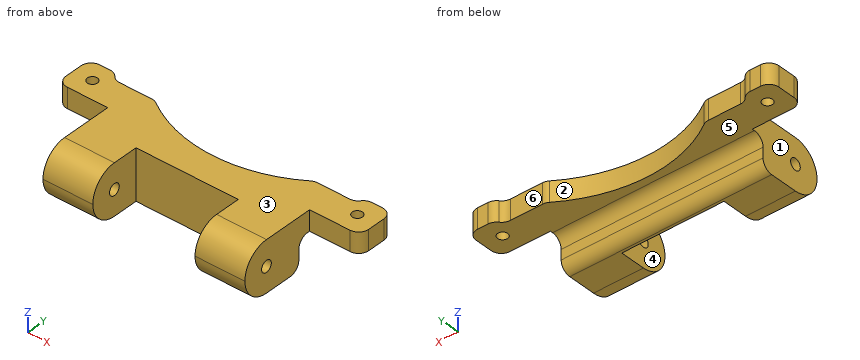
from build123d import *

# Parameters (mm, degrees)
SKETCH1_W           = 80
SKETCH1_H           = 20
BOSS_EXTRUDE1_DEPTH = 30
SKETCH2_W           = 40.5
SKETCH2_H           = 20
CUT_EXTRUDE1_DEPTH  = 20
SKETCH3_R           = 2.25
CUT_EXTRUDE2_DEPTH  = 88.749643874
FILLET1_R           = 10
SKETCH4_W           = 120
SKETCH4_H           = 20
BOSS_EXTRUDE2_DEPTH = 120
SKETCH7_R           = 2
SKETCH7_W           = 96
SKETCH7_H           = 96
CUT_EXTRUDE5_DEPTH  = 182.383571472
SKETCH8_W           = 120
SKETCH8_H           = 125
CUT_EXTRUDE6_DEPTH  = 12
FILLET2_R           = 4
FILLET3_R           = 4
SKETCH10_W          = 120
SKETCH10_H          = 105
CUT_EXTRUDE7_DEPTH  = 181.676506497
SKETCH11_R          = 55
CUT_EXTRUDE8_DEPTH  = 111.313190508
FILLET6_R           = 4
FILLET7_R           = 4


# Some blends are built 0.0001 mm under size
with BuildPart() as part:
    # Sketch1 → Boss-Extrude1 (new body)
    with BuildSketch(Plane(origin=(0, 0, 0), x_dir=(1, 0, 0), z_dir=(0, 1, 0))):
        with Locations((40, -10)):
            Rectangle(SKETCH1_W, SKETCH1_H)
    extrude(amount=BOSS_EXTRUDE1_DEPTH)

    # Sketch2 → Cut-Extrude1 (cut)
    with BuildSketch(Plane(origin=(0, 0, 0), x_dir=(-1, 0, 0), z_dir=(0, -1, 0))):
        with Locations((-40, -10)):
            Rectangle(SKETCH2_W, SKETCH2_H)
    extrude(amount=-CUT_EXTRUDE1_DEPTH, mode=Mode.SUBTRACT)

    # Sketch3 → Cut-Extrude2 (cut, through all)
    with BuildSketch(Plane.ZY):
        with Locations((10, 10)):
            Circle(SKETCH3_R)
    extrude(amount=-CUT_EXTRUDE2_DEPTH, mode=Mode.SUBTRACT)

    # Fillet1
    fillet1_edges = [part.edges().sort_by_distance(p)[0] for p in [
        (70.125, 0, 20),
        (70.125, 0, 0),
        (9.875, 0, 20),
        (9.875, 0, 0),
    ]]
    fillet(fillet1_edges, radius=FILLET1_R - 0.0001)  # a hair under: the kernel refuses the full size

    # Sketch4 → Boss-Extrude2 (add)
    with BuildSketch(Plane(origin=(0, 30, 0), x_dir=(1, 0, 0), z_dir=(0, 1, 0))):
        with Locations((40, -10)):
            Rectangle(SKETCH4_W, SKETCH4_H)
    extrude(amount=BOSS_EXTRUDE2_DEPTH)

    # Sketch7 → Cut-Extrude5 (cut, through all)
    with BuildSketch(Plane(origin=(0, 0, 0), x_dir=(-1, 0, 0), z_dir=(0, 0, -1))):
        with Locations((-92.5, 37.5)):
            Circle(SKETCH7_R)
        with Locations((12.5, 37.5)):
            Circle(SKETCH7_R)
        with Locations((12.5, 142.5)):
            Circle(SKETCH7_R)
        with Locations((-92.5, 142.5)):
            Circle(SKETCH7_R)
        with Locations((-40, 90)):
            Rectangle(SKETCH7_W, SKETCH7_H)
    extrude(amount=-CUT_EXTRUDE5_DEPTH, mode=Mode.SUBTRACT)

    # Sketch8 → Cut-Extrude6 (cut)
    with BuildSketch(Plane(origin=(0, 0, 0), x_dir=(-1, 0, 0), z_dir=(0, 0, -1))):
        with Locations((-40, 87.5)):
            Rectangle(SKETCH8_W, SKETCH8_H)
    extrude(amount=-CUT_EXTRUDE6_DEPTH, mode=Mode.SUBTRACT)

    # Fillet2
    fillet2_edges = [part.edges().sort_by_distance(p)[0] for p in [
        (40, 25, 12),
    ]]
    fillet(fillet2_edges, radius=FILLET2_R)

    # Fillet3
    fillet3_edges = [part.edges().sort_by_distance(p)[0] for p in [
        (40, 25, 0),
    ]]
    fillet(fillet3_edges, radius=FILLET3_R)

    # Sketch10 → Cut-Extrude7 (cut, through all)
    with BuildSketch(Plane(origin=(0, 0, 12), x_dir=(-1, 0, 0), z_dir=(0, 0, -1))):
        with Locations((-40, 97.5)):
            Rectangle(SKETCH10_W, SKETCH10_H)
    extrude(amount=-CUT_EXTRUDE7_DEPTH, mode=Mode.SUBTRACT)

    # Sketch11 → Cut-Extrude8 (cut, through all)
    with BuildSketch(Plane(origin=(0, 0, 12), x_dir=(-1, 0, 0), z_dir=(0, 0, -1))):
        with Locations((-40, 87)):
            Circle(SKETCH11_R)
    extrude(amount=-CUT_EXTRUDE8_DEPTH, mode=Mode.SUBTRACT)

    # Fillet6
    # the kernel refuses this fillet: 4 mm, written as the material it takes off along each edge
    with BuildSketch(Plane(origin=(-20, 30, 2), x_dir=(0, 1, 0), z_dir=(0, 0, 1)), Plane(origin=(100, 45, 2), x_dir=(0, -1, 0), z_dir=(0, 0, 1)), Plane(origin=(-20, 45, 2), x_dir=(1, 0, 0), z_dir=(0, 0, 1))) as fillet6_piece_1:
        with BuildLine():
            CenterArc((FILLET6_R, -FILLET6_R), FILLET6_R, 90, 90)
            Line((0, -FILLET6_R), (-FILLET6_R * 0.02, -FILLET6_R))
            Line((-FILLET6_R * 0.02, -FILLET6_R), (-FILLET6_R * 0.02, FILLET6_R * 0.02))
            Line((-FILLET6_R * 0.02, FILLET6_R * 0.02), (FILLET6_R, FILLET6_R * 0.02))
            Line((FILLET6_R, FILLET6_R * 0.02), (FILLET6_R, 0))
        make_face()
    extrude(amount=28, mode=Mode.SUBTRACT)
    with BuildSketch(Plane(origin=(100, 30, 30), x_dir=(-1, 0, 0), z_dir=(0, 0, -1))) as fillet6_piece_2:
        with BuildLine():
            CenterArc((FILLET6_R, FILLET6_R), FILLET6_R, 180, 90)
            Line((0, FILLET6_R), (-FILLET6_R * 0.02, FILLET6_R))
            Line((-FILLET6_R * 0.02, FILLET6_R), (-FILLET6_R * 0.02, -FILLET6_R * 0.02))
            Line((-FILLET6_R * 0.02, -FILLET6_R * 0.02), (FILLET6_R, -FILLET6_R * 0.02))
            Line((FILLET6_R, -FILLET6_R * 0.02), (FILLET6_R, 0))
        make_face()
    extrude(amount=28, mode=Mode.SUBTRACT)
    with BuildSketch(Plane(origin=(88, 45, 29.682458366), x_dir=(1, 0, 0), z_dir=(0, 0, -1))) as fillet6_piece_3:
        with BuildLine():
            CenterArc((3.872983346, 4), FILLET6_R, 194.477512186, 75.522487814)
            Line((0, 3), (-0.077459667, 2.98))
            ThreePointArc((-0.077459667, 2.98), (-0.08, 1.5), (-0.08, 0))
            Line((-0.08, 0), (0, -0.08))
            Line((0, -0.08), (3.872983346, -0.08))
            Line((3.872983346, -0.08), (3.872983346, 0))
        make_face()
    extrude(amount=27.364916731, mode=Mode.SUBTRACT)
    with BuildSketch(Plane(origin=(71.622776602, 42, 23.101442122), x_dir=(1, 0, 0), z_dir=(0, 0, -1))) as fillet6_piece_4:
        with BuildLine():
            CenterArc((1.240576849, 4), FILLET6_R, 236.151006115, 33.848993885)
            Line((-0.987447114, 0.677966102), (-1.032007593, 0.611525424))
            ThreePointArc((-1.032007593, 0.611525424), (-0.537159223, 0.275719676), (-0.045996766, -0.065454545))
            Line((-0.045996766, -0.065454545), (0, -0.08))
            Line((0, -0.08), (1.240576849, -0.08))
            Line((1.240576849, -0.08), (1.240576849, 0))
        make_face()
    extrude(amount=14.202884243, mode=Mode.SUBTRACT)
    with BuildSketch(Plane(origin=(8.377223398, 42, 23.101442122), x_dir=(0.8243940217834806, -0.5660163397355751, 0), z_dir=(0, 0, -1))) as fillet6_piece_5:
        with BuildLine():
            CenterArc((1.241341221, 3.999762854), FILLET6_R, 235.527102444, 33.848993885)
            Line((-1.022724138, 0.702186767), (-1.068005445, 0.636235245))
            Line((-1.068005445, 0.636235245), (-0.045281307, -0.065951522))
            Line((-0.045281307, -0.065951522), (0.000871117, -0.079995257))
            ThreePointArc((0.000871117, -0.079995257), (0.598892695, -0.076739245), (1.196914272, -0.079995257))
            Line((1.196914272, -0.079995257), (1.197785389, 0))
        make_face()
    extrude(amount=14.202884243, mode=Mode.SUBTRACT)
    with BuildSketch(Plane(origin=(-8, 45, 2.317541634), x_dir=(0, -1, 0), z_dir=(0, 0, 1))) as fillet6_piece_6:
        with BuildLine():
            CenterArc((4, -3.872983346), FILLET6_R, 104.477512186, 75.522487814)
            Line((0, -3.872983346), (-0.08, -3.872983346))
            Line((-0.08, -3.872983346), (-0.08, 0))
            Line((-0.08, 0), (0, 0.08))
            ThreePointArc((0, 0.08), (1.5, 0.08), (2.98, 0.077459667))
            Line((2.98, 0.077459667), (3, 0))
        make_face()
    extrude(amount=27.364916731, mode=Mode.SUBTRACT)

    # Fillet7
    fillet7_edges = [part.edges().sort_by_distance(p)[0] for p in [
        (88, 42, 16),
        (-8, 42, 16),
    ]]
    fillet(fillet7_edges, radius=FILLET7_R)


solid = part.part
CAD build for the part. Positions are in the model's coordinates, mm. Face numbers are marked on the shaded views. A direction names the side the tool comes from. Round coordinates to 2 decimals unless told otherwise and drop trailing zeros. Write each loop counter-clockwise with the first axis right and the second up, starting at its lowest first coordinate (ties: lowest second). Pieces come first, ordered by that corner, then holes. Notation, with made-up numbers: M 40,45 L 64,45 A10 ccw 64,58 Z; hole C -17.5,49.5 d8. An arc over 180 degrees is marked long. Put each result on its own line as item: value. Start each with the question number.
1) Pull direction X, two halves, no side cores. Call the marked faces 1, 2 and 3: pulls with the +X half, pulls with the -X half, needs draft (parallel to the pull), parting line crosses it, or undercut.
2) Saw through at D-D, the plane y = 37.5. Write the cut outline in (x, z), and give its area (3 significant figures).
3) Saw through at C-C, the plane z = 14.75. Write the cut outline in (x, y).
4) Pin check, flat tips, straight feed: pin 1 Ø4 at (x, z) = (21, 5) entering from -Y; pin 2 Ø3 at (x, y) = (92.5, 37.5) entering from -Z; pin 3 Ø9 at (x, z) = (87.5, 17) entering from -Y; pin 4 Ø1.5 at (x, y) = (40, 31) entering from -Z. Stop position of each tip, or through.
5) 3-axis set-ups, long thin cutter, end or side, ignore diameter. For the marked faces 4, 5 and 6: which of +Z, -Z, +X, -X, +Y, -Y reach the whole face in a straight line?
6) Drill centre lines: probe 1 along X at (y, z) = (17, 1.5); probe 2 along Y at (x, z) = (92.5, 16.75); probe 3 along X at (y, z) = (26, 12). Where is each one in solid material? Low to high. Write a range as [from, to].
7) Saw through at A-A, the plane y = 5. Write the cut outline in (x, z).
Resolved:
1. face 1: pulls with the -X half
1. face 2: undercut
1. face 3: needs draft
2. outline: M -20,12 L -14.5,12 L -14.5,20 L -20,20 Z; M -10.5,12 L 16.03,12 L 16.03,20 L -10.5,20 Z; M 63.97,12 L 90.5,12 L 90.5,20 L 63.97,20 Z; M 94.5,12 L 100,12 L 100,20 L 94.5,20 Z
2. area: 512 mm²
3. outline: M -20,34 A4 ccw -16,30 L 0,30 L 0,1.2 L 19.75,1.2 L 19.75,20 L 60.25,20 L 60.25,1.2 L 80,1.2 L 80,30 L 96,30 A4 ccw 100,34 L 100,41 A4 ccw 96,45 L 91.87,45 A4 ccw 88.75,43.5 A4 cw 85.63,42 L 72.86,42 A4 ccw 70.64,41.32 A55 cw 9.36,41.32 A4 ccw 7.14,42 L -5.63,42 A4 cw -8.75,43.5 A4 ccw -11.87,45 L -16,45 A4 ccw -20,41 Z; hole C -12.5,37.5 d4; hole C 92.5,37.5 d4
4. pin 1: y = 0.61
4. pin 2: through
4. pin 3: y = 30
4. pin 4: z = 12
5. face 4: +Z, -Z, -Y
5. face 5: -Z, +X, -X, +Y
5. face 6: +Z, -Z, +Y
6. probe 1: [0, 19.75], [60.25, 80]
6. probe 2: [30, 35.5], [39.5, 45]
6. probe 3: [0, 80]
7. outline: M 0,1.34 L 19.75,1.34 L 19.75,18.66 L 0,18.66 Z; M 60.25,1.34 L 80,1.34 L 80,18.66 L 60.25,18.66 Z
